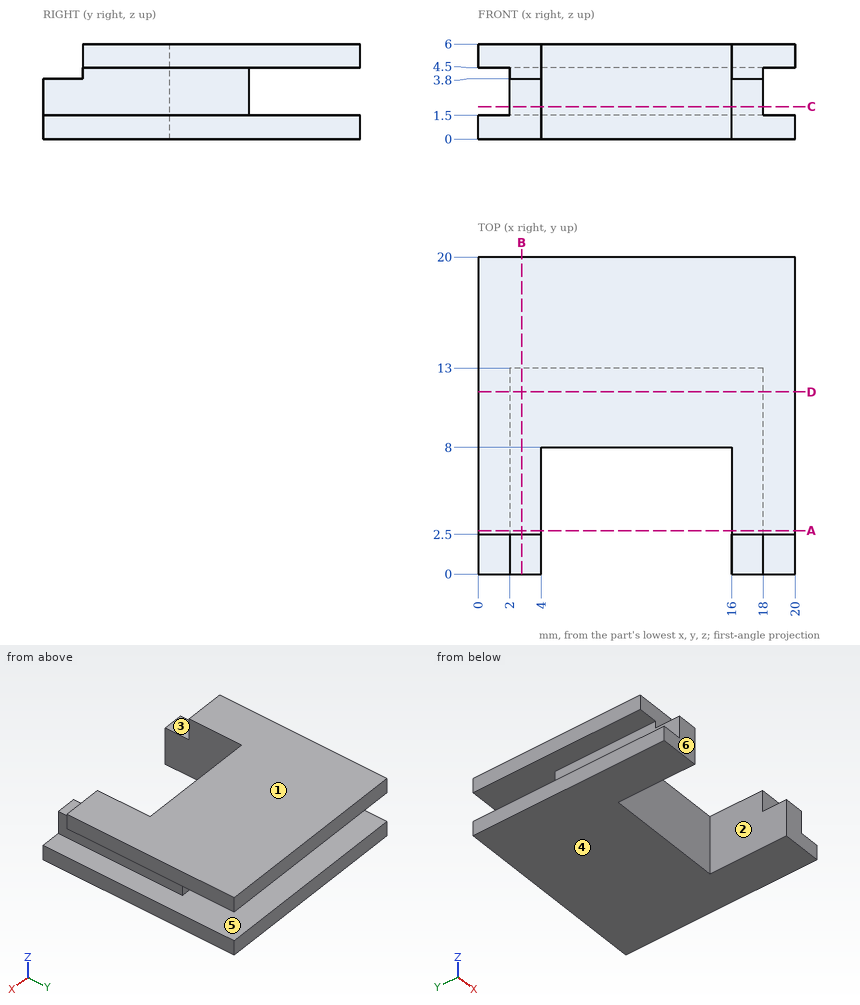
Geometry check sheet. Reference: drawing and pictorial views, mm from the part's lowest x, y, z. A direction names the side the tool comes from. Coordinates: 2 decimals unless noted, no trailing zeros. Write each loop counter-clockwise with the first axis right and the second up, starting at its lowest first coordinate (ties: lowest second). Pieces come first, ordered by that corner, then holes. Notation, with made-up numbers: (46.5, 12) -> (87.5, 12) arc R28 ccw to (87.5, 43) -> close; hole circle Ø9 at (-13, 18.5). An arc over 180 degrees is marked (long way). Use a Markdown table: item, result.
1. Sectioned sample at B-B (x = 2.75). Enter the section's corners in (y, z), plus the area to 3 significant figures.
Reported:
| item | result |
|---|---|
| outline | (0, 0) -> (20, 0) -> (20, 1.5) -> (13, 1.5) -> (13, 4.5) -> (20, 4.5) -> (20, 6) -> (2.5, 6) -> (2.5, 3.8) -> (0, 3.8) -> close |
| area | 93.5 mm2 |
2. Tool access check on the marked faces 1, 2 and 3. Record the directions out of +Z, -Z, +X, -X, +Y, -Y that give a thin tool (end or side, any length) a straight path to the whole face; none if there is none.
Reported:
| item | result |
|---|---|
| face 1 | +Z, +X, -X, +Y, -Y |
| face 2 | +Z, -Z, -Y |
| face 3 | +Z, +X, -X, -Y |
3. Go/stop test with flat-tipped pins: pin 1 Ø1 at (x, y) = (16.5, 1.5) entering from +Z; pin 2 Ø1.5 at (y, z) = (5, 3.5) entering from -X. Record where each tip stops, or that it passes through.
Reported:
| item | result |
|---|---|
| pin 1 | stops at z = 3.8 |
| pin 2 | stops at x = 2 |
4. Sectioned sample at A-A (y = 2.75). Enter the section's corners in (x, z).
Reported:
| item | result |
|---|---|
| outline | (0, 0) -> (4, 0) -> (4, 6) -> (0, 6) -> (0, 4.5) -> (2, 4.5) -> (2, 1.5) -> (0, 1.5) -> close; (16, 0) -> (20, 0) -> (20, 1.5) -> (18, 1.5) -> (18, 4.5) -> (20, 4.5) -> (20, 6) -> (16, 6) -> close |
5. Sectioned sample at C-C (z = 2.05). Enter the section's corners in (x, y), plus the area to 3 significant figures.
Reported:
| item | result |
|---|---|
| outline | (2, 0) -> (4, 0) -> (4, 8) -> (16, 8) -> (16, 0) -> (18, 0) -> (18, 13) -> (2, 13) -> close |
| area | 112 mm2 |
6. Scan lines: line 1 along X through (y, z) = (1, 0.35); line 2 along Z through (x, y) = (15.75, 19); line 3 along X through (y, z) = (9.75, 2.6). Record each from-to range of solid material in increasing order.
Reported:
| item | result |
|---|---|
| line 1 | x = 0 to 4, 16 to 20 |
| line 2 | z = 0 to 1.5, 4.5 to 6 |
| line 3 | x = 2 to 18 |
7. Sectioned sample at D-D (y = 11.5). Enter the section's corners in (x, z).
Reported:
| item | result |
|---|---|
| outline | (0, 0) -> (20, 0) -> (20, 1.5) -> (18, 1.5) -> (18, 4.5) -> (20, 4.5) -> (20, 6) -> (0, 6) -> (0, 4.5) -> (2, 4.5) -> (2, 1.5) -> (0, 1.5) -> close |
8. Release check for a two-part mould opening along Z. For the marked faces 4, 5 and 6 record: pulls with the +Z half, pulls with the -Z half, needs draft (parallel to the pull), parting line crosses it, or undercut.
Reported:
| item | result |
|---|---|
| face 4 | pulls with the -Z half |
| face 5 | undercut |
| face 6 | needs draft |
